Could you check a few things on this model? Use its own coordinates, in mm. A direction names the side the tool comes from. Give positions to 0.01 mm unless a question says otherwise; leave off trailing zeros. Order: outer loops, then holes, each group sorted by start corner. A loop starts at its lowest first (then second) coordinate and runs counter-clockwise, first axis right, second up.
from build123d import *

# Parameters (mm, degrees)
SKETCH1_R                = 20
BOSS_EXTRUDE1_DEPTH      = 10
CUT_EXTRUDE1_DEPTH       = 31
BOSS_EXTRUDE2_DEPTH      = 10
SKETCH5_R                = 12.5
BOSS_EXTRUDE3_DEPTH      = 6
BOSS_EXTRUDE4_DEPTH      = 10
BOSS_EXTRUDE4_DEPTH_BACK = 20
SKETCH7_R                = 2.5
CUT_EXTRUDE2_DEPTH       = 97.465771152
BOSS_EXTRUDE5_DEPTH      = 2.5
CUT_EXTRUDE3_START       = -2.5
SKETCH9_R                = 12.5
CUT_EXTRUDE3_DEPTH       = 2.5
SKETCH10_W               = 45
SKETCH10_H               = 15
BOSS_EXTRUDE6_DEPTH      = 9.95
SKETCH11_W               = 45
SKETCH11_H               = 15
BOSS_EXTRUDE7_DEPTH      = 9.95
SKETCH12_R               = 47.5
CUT_EXTRUDE4_DEPTH       = 10


with BuildPart() as part:
    # Sketch1 → Boss-Extrude1 (new body)
    with BuildSketch(Plane(origin=(0, 0, 0), x_dir=(1, 0, 0), z_dir=(0, 1, 0))):
        with Locations(Location((0, 0, 0), (0, 0, 270))):
            Circle(SKETCH1_R)
    extrude(amount=BOSS_EXTRUDE1_DEPTH)

    # Sketch2 → Cut-Extrude1 (cut, through all)
    with BuildSketch(Plane(origin=(0, 10, 0), x_dir=(1, 0, 0), z_dir=(0, 1, 0))):
        with BuildLine():
            Line((1.962141687, 3.6), (-1.962141687, 3.6))
            ThreePointArc((-1.962141687, 3.6), (-3.686980014, 1.793370675), (-4.043407712, -0.678862337))
            ThreePointArc((-4.043407712, -0.678862337), (-2.899137803, -2.899137803), (-0.678862337, -4.043407712))
            ThreePointArc((-0.678862337, -4.043407712), (1.793370675, -3.686980014), (3.6, -1.962141687))
            Line((3.6, -1.962141687), (3.6, 1.962141687))
            ThreePointArc((3.6, 1.962141687), (2.899137803, 2.899137803), (1.962141687, 3.6))
        make_face()
    extrude(amount=-CUT_EXTRUDE1_DEPTH, mode=Mode.SUBTRACT)

    # Sketch3 → Boss-Extrude2 (add)
    with BuildSketch(Plane(origin=(0, 0, 0), x_dir=(1, 0, 0), z_dir=(0, 1, 0))):
        with BuildLine():
            Line((-17.5, 59.682458366), (-17.5, 9.682458366))
            ThreePointArc((-17.5, 9.682458366), (0, 20), (17.5, 9.682458366))
            Line((17.5, 9.682458366), (17.5, 59.682458366))
            Line((17.5, 59.682458366), (-17.5, 59.682458366))
        make_face()
    extrude(amount=BOSS_EXTRUDE2_DEPTH)

    # Sketch5 → Boss-Extrude3 (add)
    with BuildSketch(Plane.XZ):
        with Locations(Location((0, 0, 0), (0, 0, 90))):
            Circle(SKETCH5_R)
        with BuildLine():
            Line((3.6, 1.962141687), (3.6, -1.962141687))
            ThreePointArc((3.6, -1.962141687), (2.899137803, -2.899137803), (1.962141687, -3.6))
            Line((1.962141687, -3.6), (-1.962141687, -3.6))
            ThreePointArc((-1.962141687, -3.6), (-2.899137803, 2.899137803), (3.6, 1.962141687))
        make_face(mode=Mode.SUBTRACT)
    extrude(amount=BOSS_EXTRUDE3_DEPTH)

    # Sketch6 → Boss-Extrude4 (add, two sides: drawn at the far end of the back side and taken through both)
    with BuildSketch(Plane(origin=(0, 0, -59.682458366), x_dir=(-1, 0, 0), z_dir=(0, 0, -1)).offset(-BOSS_EXTRUDE4_DEPTH_BACK)):
        Polygon((-32.5, 10), (32.5, 10), (32.5, -15), (22.5, -15), (22.5, 0), (-22.5, 0), (-22.5, -15), (-32.5, -15), align=None)
    extrude(amount=BOSS_EXTRUDE4_DEPTH + BOSS_EXTRUDE4_DEPTH_BACK)

    # Sketch7 → Cut-Extrude2 (cut, through all)
    with BuildSketch(Plane(origin=(32.5, 0, 0), x_dir=(0, 0, -1), z_dir=(1, 0, 0))):
        with Locations(Location((54.682458366, -7.5, 0), (0, 0, 90))):
            Circle(SKETCH7_R)
    extrude(amount=-CUT_EXTRUDE2_DEPTH, mode=Mode.SUBTRACT)

    # Sketch8 → Boss-Extrude5 (add)
    with BuildSketch(Plane(origin=(0, 10, 0), x_dir=(1, 0, 0), z_dir=(0, 1, 0))):
        with BuildLine():
            Line((-32.5, 69.682458366), (-32.5, 39.682458366))
            Line((-32.5, 39.682458366), (-17.5, 39.682458366))
            Line((-17.5, 39.682458366), (-17.5, 9.682458366))
            ThreePointArc((-17.5, 9.682458366), (0, -20), (17.5, 9.682458366))
            Line((17.5, 9.682458366), (17.5, 39.682458366))
            Line((17.5, 39.682458366), (32.5, 39.682458366))
            Line((32.5, 39.682458366), (32.5, 69.682458366))
            Line((32.5, 69.682458366), (-32.5, 69.682458366))
        make_face()
    extrude(amount=BOSS_EXTRUDE5_DEPTH)

    # Sketch9 → Cut-Extrude3 (cut)
    with BuildSketch(Plane.XZ.offset(6).offset(CUT_EXTRUDE3_START)):
        with Locations(Location((0, 0, 0), (0, 0, 90))):
            Circle(SKETCH9_R)
    extrude(amount=CUT_EXTRUDE3_DEPTH, mode=Mode.SUBTRACT)

    # Sketch10 → Boss-Extrude6 (add)
    with BuildSketch(Plane(origin=(0, 0, -69.682458366), x_dir=(-1, 0, 0), z_dir=(0, 0, -1))):
        with Locations((0, -7.5)):
            Rectangle(SKETCH10_W, SKETCH10_H)
    extrude(amount=-BOSS_EXTRUDE6_DEPTH)

    # Sketch11 → Boss-Extrude7 (add)
    with BuildSketch(Plane.XY.offset(-39.682458366)):
        with Locations((0, -7.5)):
            Rectangle(SKETCH11_W, SKETCH11_H)
    extrude(amount=-BOSS_EXTRUDE7_DEPTH)

    # Sketch12 → Cut-Extrude4 (cut)
    with BuildSketch(Plane(origin=(0, 0, -69.682458366), x_dir=(-1, 0, 0), z_dir=(0, 0, -1))):
        with Locations((0, -60)):
            Circle(SKETCH12_R)
    extrude(amount=-CUT_EXTRUDE4_DEPTH, mode=Mode.SUBTRACT)


solid = part.part
Item 1: Imagine slicing it at C-C on z = 3. List the corners of the cut face in (x, y) for me.
Findings:
outline: (-19.77, 0) - (-12.13, 0) - (-12.13, -3.5) - (-2.79, -3.5) - (-2.79, 10) - (2.79, 10) - (2.79, -3.5) - (12.13, -3.5) - (12.13, 0) - (19.77, 0) - (19.77, 12.5) - (-19.77, 12.5) - close
Item 2: Please list where these lines run through material, in increasing order: line 1 along X through (y, z) = (-1.7, 0); line 2 along Z through (x, y) = (28.75, -7.5); line 3 along X through (y, z) = (-3, -56.5).
Findings:
line 1: x = -12.5 to -4.1, 3.6 to 12.5
line 2: z = -69.68 to -57.18, -52.18 to -39.68
line 3: x = -32.5 to -22.5, 22.5 to 32.5
Item 3: Imagine slicing it at A-A on y = -7.5. List the corners of the cut face in (x, z) for me, then the cut area to 3 significant figures.
Findings:
outline: (-32.5, -69.68) - (32.5, -69.68) - (32.5, -57.18) - (22.5, -57.18) - (22.5, -59.73) - (-22.5, -59.73) - (-22.5, -57.18) - (-32.5, -57.18) - close; (-32.5, -52.18) - (-22.5, -52.18) - (-22.5, -49.63) - (22.5, -49.63) - (22.5, -52.18) - (32.5, -52.18) - (32.5, -39.68) - (-32.5, -39.68) - close
area: 1,400 mm2
Item 4: Imagine slicing it at D-D on z = -35. List the corners of the cut face in (x, y) for me.
Findings:
outline: (-17.5, 0) - (17.5, 0) - (17.5, 12.5) - (-17.5, 12.5) - close
Item 5: For faces 4 (the cylindrical face through (-0.2, -12.5, -64.8)), 5 (the flat face through (17.5, 6, -24)), 6 (the flat face through (0, -7, -59.732)), 7 (the flat face through (-17.5, 6, -25)), which set-ups out of +Z, -Z, +X, -X, +Y, -Y let a thin tool reach every point of the face, with its end or its side?
Findings:
face 4: -Z, -Y
face 5: +X, +Y, -Y
face 6: -Y
face 7: -X, +Y, -Y
Item 6: We'd pull the mould along Y, two halves only. Please class faces 1 (the flat face through (0, -1, -69.682)), 2 (the flat face through (0, -15, -48)), 3 (the cylindrical face through (27.57, -8.042, -57.123)): +Y half, -Y half, draft (parallel to the pull), parting line (faces both ways), or undercut.
Findings:
face 1: draft
face 2: -Y half
face 3: undercut
Item 7: For pin 1 (8 mm diameter, centred on x = 7, z = -55, fed in from -Y); pin 2 (20 mm diameter, centred on x = 9, z = -6, fed in from -Y); pin 3 (3 mm diameter, centred on x = 0.5, y = 3.5, fed in from +Z), each with a flat end and sliding along its axis, tell me the tip position at first contact or that it passes through.
Findings:
pin 1: stops at y = 0
pin 2: stops at y = -3.5
pin 3: stops at z = 20
Item 8: Imagine slicing it at B-B on x = -21.5. List the corners of the cut face in (y, z) for me.
Findings:
outline: (-15, -69.68) - (12.5, -69.68) - (12.5, -39.68) - (-15, -39.68) - (-15, -49.63) - (0, -49.63) - (0, -59.73) - (-15, -59.73) - close
